Geometry check sheet. Reference: the model listing, model coordinates, mm. A direction names the side the tool comes from. Give positions to 0.01 mm unless a question says otherwise; leave off trailing zeros. Order: outer loops, then holes, each group sorted by start corner. A loop starts at its lowest first (then second) coordinate and runs counter-clockwise, first axis right, second up.
from build123d import *

# Parameters (mm, degrees)
ESQUISSE1_W        = 4
ESQUISSE1_H        = 29
BOSS_EXTRU_2_DEPTH = 3


with BuildPart() as part:
    # Esquisse1 → Boss.-Extru.2 (new body)
    with BuildSketch(Plane.XY):
        Polygon((-35, 0), (-35, 8), (-25, 18), (-15, 8), (-15, 0), (0, 0), (0, 35), (-50, 35), (-50, 0), align=None)
        with Locations((-10, 17.5)):
            Rectangle(ESQUISSE1_W, ESQUISSE1_H, mode=Mode.SUBTRACT)
        with Locations((-40, 17.5)):
            Rectangle(ESQUISSE1_W, ESQUISSE1_H, mode=Mode.SUBTRACT)
    extrude(amount=BOSS_EXTRU_2_DEPTH)


solid = part.part
Item 1: Sectioned sample at A-A (y = 13). Enter the section's corners in (x, z).
Reported:
outline: (-50, 0) - (-42, 0) - (-42, 3) - (-50, 3) - close; (-38, 0) - (-30, 0) - (-30, 3) - (-38, 3) - close; (-20, 0) - (-12, 0) - (-12, 3) - (-20, 3) - close; (-8, 0) - (0, 0) - (0, 3) - (-8, 3) - close
Item 2: Gauge pin test, flat end, axial feed: pin 1 (3 mm diameter, centred on x = -41, y = 24, fed in from -Z). Record the tip position at first contact, or that the pin passes through.
Reported:
pin 1: stops at z = 0
Item 3: Sectioned sample at D-D (x = -22.5). Enter the section's corners in (y, z).
Reported:
outline: (15.5, 0) - (35, 0) - (35, 3) - (15.5, 3) - close
Item 4: Sectioned sample at C-C (z = 1.4). Enter the section's corners in (x, y), and give its area (3 significant figures).
Reported:
outline: (-50, 0) - (-35, 0) - (-35, 8) - (-25, 18) - (-15, 8) - (-15, 0) - (0, 0) - (0, 35) - (-50, 35) - close; hole (-42, 3) - (-38, 3) - (-38, 32) - (-42, 32) - close; hole (-12, 3) - (-8, 3) - (-8, 32) - (-12, 32) - close
area: 1,260 mm2
Item 5: Scan lines: L1, parallel to X at y = 19, z = 2.1; L2, parallel to X at y = 2, z = 1.1; L3, parallel to X at y = 14.5, z = 2.65. Record each from-to range of solid material in increasing order.
Reported:
L1: x = -50 to -42, -38 to -12, -8 to 0
L2: x = -50 to -35, -15 to 0
L3: x = -50 to -42, -38 to -28.5, -21.5 to -12, -8 to 0
Item 6: Sectioned sample at B-B (y = 26). Enter the section's corners in (x, z), and give its area (3 significant figures).
Reported:
outline: (-50, 0) - (-42, 0) - (-42, 3) - (-50, 3) - close; (-38, 0) - (-12, 0) - (-12, 3) - (-38, 3) - close; (-8, 0) - (0, 0) - (0, 3) - (-8, 3) - close
area: 126 mm2
Item 7: Set-up check for faces 1 (the flat face through (0, 17, 1)), 2 (the flat face through (-15, 4, 1)), 3 (the flat face through (-40, 32, 1)): record each of +Z, -Z, +X, -X, +Y, -Y from which the full face is reachable in a straight line by a thin tool's end or side.
Reported:
face 1: +Z, -Z, +X, +Y, -Y
face 2: +Z, -Z, -Y
face 3: +Z, -Z
